from build123d import *

# Parameters (mm, degrees)
IZIM1_R             = 2.5
BOSS_EXTRUDE1_DEPTH = 350


with BuildPart() as part:
    # Çizim1 → Boss-Extrude1 (new body)
    with BuildSketch(Plane(origin=(0, 0, 0), x_dir=(0, 0, -1), z_dir=(1, 0, 0))):
        with BuildLine():
            Line((-9.5, 10), (-4.65, 10))
            Line((-4.65, 10), (-4.65, 9.8))
            Line((-4.65, 9.8), (-4.2, 9.8))
            Line((-4.2, 9.8), (-4.2, 8.2))
            Line((-4.2, 8.2), (-5.65, 8.2))
            Line((-5.65, 8.2), (-5.65, 6.857106781))
            ThreePointArc((-5.65, 6.857106781), (-5.611939766, 6.665765065), (-5.503553391, 6.503553391))
            Line((-5.503553391, 6.503553391), (-3.146446609, 4.146446609))
            ThreePointArc((-3.146446609, 4.146446609), (-2.984234935, 4.038060234), (-2.792893219, 4))
            Line((-2.792893219, 4), (2.792893219, 4))
            ThreePointArc((2.792893219, 4), (2.984234935, 4.038060234), (3.146446609, 4.146446609))
            Line((3.146446609, 4.146446609), (5.503553391, 6.503553391))
            ThreePointArc((5.503553391, 6.503553391), (5.611939766, 6.665765065), (5.65, 6.857106781))
            Line((5.65, 6.857106781), (5.65, 8.2))
            Line((5.65, 8.2), (4.2, 8.2))
            Line((4.2, 8.2), (4.2, 9.8))
            Line((4.2, 9.8), (4.65, 9.8))
            Line((4.65, 9.8), (4.65, 10))
            Line((4.65, 10), (9.5, 10))
            ThreePointArc((9.5, 10), (9.853553391, 9.853553391), (10, 9.5))
            Line((10, 9.5), (10, 4.65))
            Line((10, 4.65), (9.8, 4.65))
            Line((9.8, 4.65), (9.8, 4.2))
            Line((9.8, 4.2), (8.2, 4.2))
            Line((8.2, 4.2), (8.2, 5.65))
            Line((8.2, 5.65), (6.857106781, 5.65))
            ThreePointArc((6.857106781, 5.65), (6.665765065, 5.611939766), (6.503553391, 5.503553391))
            Line((6.503553391, 5.503553391), (4.146446609, 3.146446609))
            ThreePointArc((4.146446609, 3.146446609), (4.038060234, 2.984234935), (4, 2.792893219))
            Line((4, 2.792893219), (4, -2.792893219))
            ThreePointArc((4, -2.792893219), (4.038060234, -2.984234935), (4.146446609, -3.146446609))
            Line((4.146446609, -3.146446609), (6.503553391, -5.503553391))
            ThreePointArc((6.503553391, -5.503553391), (6.665765065, -5.611939766), (6.857106781, -5.65))
            Line((6.857106781, -5.65), (8.2, -5.65))
            Line((8.2, -5.65), (8.2, -4.2))
            Line((8.2, -4.2), (9.8, -4.2))
            Line((9.8, -4.2), (9.8, -4.65))
            Line((9.8, -4.65), (10, -4.65))
            Line((10, -4.65), (10, -9.5))
            ThreePointArc((10, -9.5), (9.853553391, -9.853553391), (9.5, -10))
            Line((9.5, -10), (4.65, -10))
            Line((4.65, -10), (4.65, -9.8))
            Line((4.65, -9.8), (4.2, -9.8))
            Line((4.2, -9.8), (4.2, -8.2))
            Line((4.2, -8.2), (5.65, -8.2))
            Line((5.65, -8.2), (5.65, -6.857106781))
            ThreePointArc((5.65, -6.857106781), (5.611939766, -6.665765065), (5.503553391, -6.503553391))
            Line((5.503553391, -6.503553391), (3.146446609, -4.146446609))
            ThreePointArc((3.146446609, -4.146446609), (2.984234935, -4.038060234), (2.792893219, -4))
            Line((2.792893219, -4), (-2.792893219, -4))
            ThreePointArc((-2.792893219, -4), (-2.984234935, -4.038060234), (-3.146446609, -4.146446609))
            Line((-3.146446609, -4.146446609), (-5.503553391, -6.503553391))
            ThreePointArc((-5.503553391, -6.503553391), (-5.611939766, -6.665765065), (-5.65, -6.857106781))
            Line((-5.65, -6.857106781), (-5.65, -8.2))
            Line((-5.65, -8.2), (-4.2, -8.2))
            Line((-4.2, -8.2), (-4.2, -9.8))
            Line((-4.2, -9.8), (-4.65, -9.8))
            Line((-4.65, -9.8), (-4.65, -10))
            Line((-4.65, -10), (-9.5, -10))
            ThreePointArc((-9.5, -10), (-9.853553391, -9.853553391), (-10, -9.5))
            Line((-10, -9.5), (-10, -4.65))
            Line((-10, -4.65), (-9.8, -4.65))
            Line((-9.8, -4.65), (-9.8, -4.2))
            Line((-9.8, -4.2), (-8.2, -4.2))
            Line((-8.2, -4.2), (-8.2, -5.65))
            Line((-8.2, -5.65), (-6.857106781, -5.65))
            ThreePointArc((-6.857106781, -5.65), (-6.665765065, -5.611939766), (-6.503553391, -5.503553391))
            Line((-6.503553391, -5.503553391), (-4.146446609, -3.146446609))
            ThreePointArc((-4.146446609, -3.146446609), (-4.038060234, -2.984234935), (-4, -2.792893219))
            Line((-4, -2.792893219), (-4, 2.792893219))
            ThreePointArc((-4, 2.792893219), (-4.038060234, 2.984234935), (-4.146446609, 3.146446609))
            Line((-4.146446609, 3.146446609), (-6.503553391, 5.503553391))
            ThreePointArc((-6.503553391, 5.503553391), (-6.665765065, 5.611939766), (-6.857106781, 5.65))
            Line((-6.857106781, 5.65), (-8.2, 5.65))
            Line((-8.2, 5.65), (-8.2, 4.2))
            Line((-8.2, 4.2), (-9.8, 4.2))
            Line((-9.8, 4.2), (-9.8, 4.65))
            Line((-9.8, 4.65), (-10, 4.65))
            Line((-10, 4.65), (-10, 9.5))
            ThreePointArc((-10, 9.5), (-9.853553391, 9.853553391), (-9.5, 10))
        make_face()
        Circle(IZIM1_R, mode=Mode.SUBTRACT)
    extrude(amount=BOSS_EXTRUDE1_DEPTH)


solid = part.part
Verification items for the finished model (mm, model axes). A direction names the side the tool comes from. Round coordinates to 2 decimals unless told otherwise and drop trailing zeros. Put each result on its own line as item: value.
1) Set-up check for faces 1 (the flat face through (173, -4, 0)), 2 (the flat face through (350, 2, 2)): record each of +Z, -Z, +X, -X, +Y, -Y from which the full face is reachable in a straight line by a thin tool's end or side.
Final values:
face 1: +X, -X, -Y
face 2: +Z, -Z, +X, +Y, -Y
2) Depth check by flat-ended pin: pin 1 (2 mm diameter, centred on x = 222.5, y = -3.5, fed in from +Z); pin 2 (2 mm diameter, centred on x = 38.5, y = 2, fed in from -Z). Enter the tip coordinate at first touch or a pass-through.
Final values:
pin 1: stops at z = 9.8
pin 2: stops at z = -4.04
3) Mould release check, pull along Y, two halves, no side actions. Record for faces 3 (the flat face through (173, 0, 4)), 4 (the flat face through (173, 0, -4)), 5 (the flat face through (0, 2, 2)), 6 (the flat face through (173, 4, 0)): +Y half, -Y half, draft (parallel to the pull), parting line (faces both ways), or undercut.
Final values:
face 3: undercut
face 4: undercut
face 5: draft
face 6: +Y half
4) Material ranges on line 1 (Z direction, x = 108.5, y = 7.75); line 2 (Y direction, x = 136.5, z = 0); line 3 (Y direction, x = 325.5, z = -8.25), recorded low to high.
Final values:
line 1: z = -10 to -5.65, 5.65 to 10
line 2: y = -4 to -2.5, 2.5 to 4
line 3: y = -10 to -4.2, 4.2 to 10
